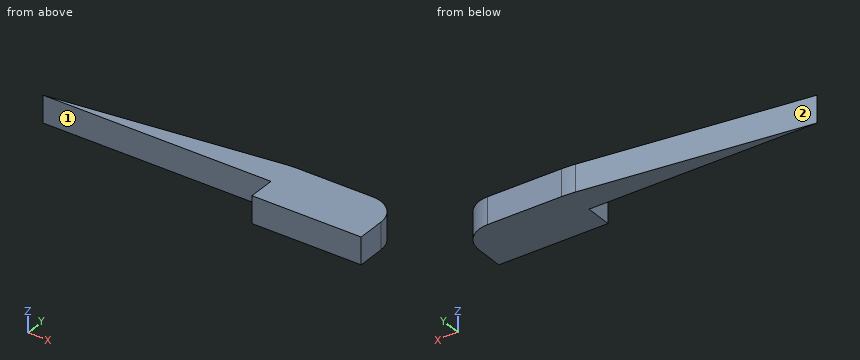
```python
from build123d import *

# Parameters (mm, degrees)
BOSS_EXTRUDE1_DEPTH = 3.175


with BuildPart() as part:
    # Sketch1 → Boss-Extrude1 (new body)
    with BuildSketch(Plane.XY):
        with BuildLine():
            Line((38.2016, 0), (38.2016, -3.2766))
            Line((38.2016, -3.2766), (25.2984, -3.2766))
            Line((25.2984, -3.2766), (25.2984, -0.1016))
            Line((25.2984, -0.1016), (-1.631925387, -0.1016))
            Line((-1.631925387, -0.1016), (24.602830345, 3.177744467))
            ThreePointArc((24.602830345, 3.177744467), (25.395214732, 3.251862215), (26.190673403, 3.2766))
            Line((26.190673403, 3.2766), (34.925, 3.2766))
            ThreePointArc((34.925, 3.2766), (37.241906079, 2.316906079), (38.2016, 0))
        make_face()
    extrude(amount=BOSS_EXTRUDE1_DEPTH)


solid = part.part
```
For this review, take the finished solid that the model builds, in its own axes (mm). Face numbers are marked on the shaded views. A direction names the side the tool comes from. Coordinates: 2 decimals unless noted, no trailing zeros. Loops run counter-clockwise (first coordinate to the right, second up) from the corner with the lowest first, then second, coordinate; pieces in that order, holes last.
1. Add section C-C, the plane x = 6.5. Give the boundary of the cut face in (y, z) (3 decimals), then the cut area to 3 significant figures.
2. For line 1 (X direction, y = -3, z = 2.8); line 2 (Y direction, x = 10.5, z = 2.55); line 3 (Y direction, x = 22, z = 0.85), list the stretches that pass through material, from the lowest coordinate up.
3. Insertion check: P1, Ø1.6, axis at y = -1.5, z = 1, coming from the -X side; P2, Ø1, axis at x = 17, z = 1.5, coming from the -Y side. Each pin has a flat end and moves straight along its axis. Give the tip position at first contact, or say it passes through.
4. Add section B-B, the plane y = -2.5. Give the boundary of the cut face in (x, z) (3 decimals), then the cut area to 3 significant figures.
5. For the marked faces 1 and 2, list the 3-axis set-ups (+Z, -Z, +X, -X, +Y, -Y) from which the entire face can be reached by the end or side of a thin tool; tool diameter is ignored.
6. Add section A-A, the plane z = 1.15. Give the boundary of the cut face in (x, y) (3 decimals), then the cut area to 3 significant figures.
Result:
1. outline: (-0.102, 0) - (0.915, 0) - (0.915, 3.175) - (-0.102, 3.175) - close
1. area: 3.23 mm2
2. line 1: x = 25.3 to 38.2
2. line 2: y = -0.1 to 1.41
2. line 3: y = -0.1 to 2.85
3. P1: stops at x = 25.3
3. P2: stops at y = -0.1
4. outline: (25.298, 0) - (38.202, 0) - (38.202, 3.175) - (25.298, 3.175) - close
4. area: 41.0 mm2
5. face 1: +Z, -Z, -X, -Y
5. face 2: +Z, -Z, -X, +Y
6. outline: (-1.632, -0.102) - (25.298, -0.102) - (25.298, -3.277) - (38.202, -3.277) - (38.202, 0) arc R3.277 ccw to (34.925, 3.277) - (26.191, 3.277) arc R12.802 ccw to (24.603, 3.178) - close
6. area: 128 mm2
